Could you check a few things on this drawing? It's one solid part, dimensions in mm from its lowest x, y, z. Give positions to 0.01 mm unless a question says otherwise; leave off trailing zeros. Order: outer loops, then holes, each group sorted by start corner. A loop starts at its lowest first (then second) coordinate and runs counter-clockwise, first axis right, second up. Notation, with made-up numbers: (37.25, 68.25) - (43.25, 68.25) arc R33 ccw to (43.25, 106.25) - close; hole circle Ø5 at (38, -15). An arc over 180 degrees is marked (long way). Return JSON: item names as keys, results as strings.
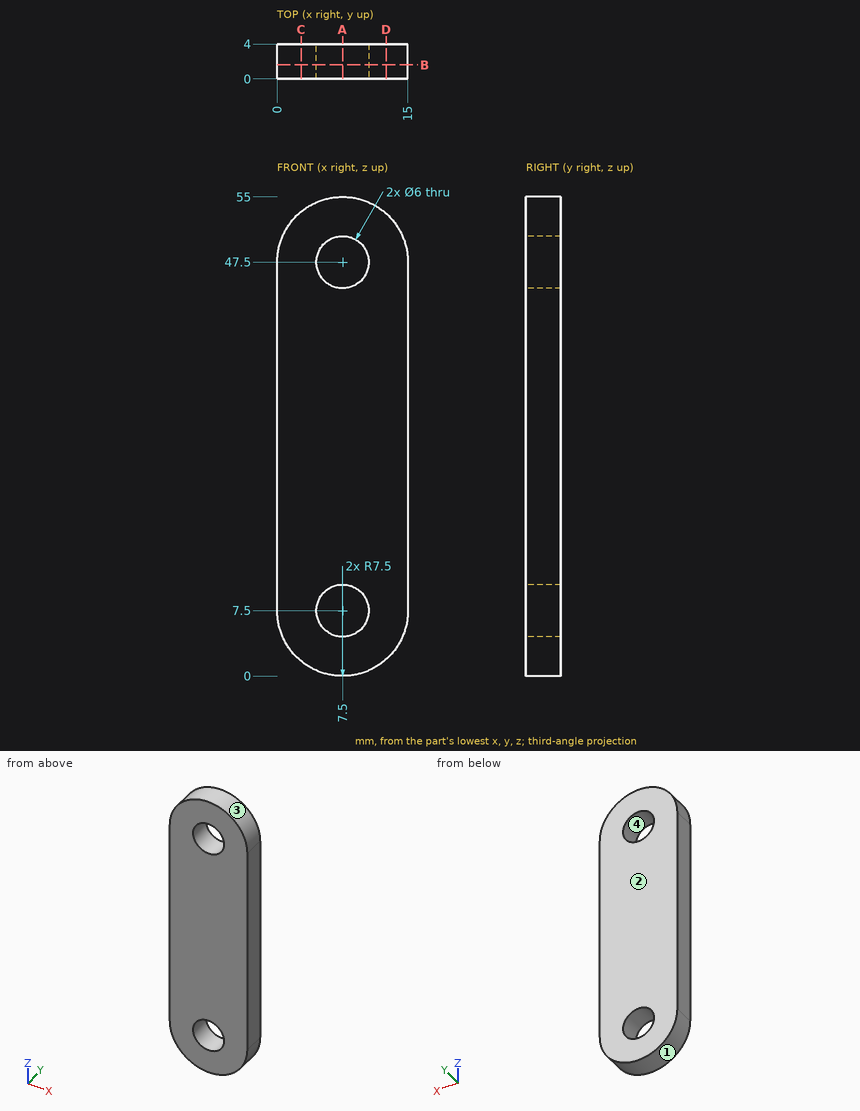
1. Suppose I cut it at D-D (x = 12.5). List the corners of the cut face in (y, z) for me.
Checks:
{"outline": "(0, 1.91) - (4, 1.91) - (4, 53.09) - (0, 53.09) - close"}
2. Suppose I cut it at A-A (x = 7.5). List the corners of the cut face in (y, z) for me, plus the area to 3 significant figures.
Checks:
{"outline": "(0, 0) - (4, 0) - (4, 4.5) - (0, 4.5) - close; (0, 10.5) - (4, 10.5) - (4, 44.5) - (0, 44.5) - close; (0, 50.5) - (4, 50.5) - (4, 55) - (0, 55) - close", "area": "172 mm^2"}
3. If I drill on L1, parallel to Z at x = 7.5, y = 3.15; L2, parallel to Z at x = 10, y = 2.65; L3, parallel to X at y = 3.85, z = 47, over which ranges is the centre line in solid material (lowest first)? Write a range as [from, to].
Checks:
{"L1": "[0, 4.5], [10.5, 44.5], [50.5, 55]", "L2": "[0.43, 5.84], [9.16, 45.84], [49.16, 54.57]", "L3": "[0, 4.54], [10.46, 15]"}
4. Thinking about a two-plate mould opening in Z: for the marked faces 1, 2, 3 and 4, which applies, +Z half, -Z half, draft (parallel to the pull), parting line (faces both ways), or undercut?
Checks:
{"face 1": "-Z half", "face 2": "draft", "face 3": "+Z half", "face 4": "undercut"}
5. Suppose I cut it at C-C (x = 2.75). List the corners of the cut face in (y, z) for me, plus the area to 3 significant figures.
Checks:
{"outline": "(0, 1.7) - (4, 1.7) - (4, 53.3) - (0, 53.3) - close", "area": "206 mm^2"}
6. Suppose I cut it at B-B (y = 1.6). List the corners of the cut face in (x, z) for me, plus the area to 3 significant figures.
Checks:
{"outline": "(0, 7.5) arc R7.5 ccw to (15, 7.5) - (15, 47.5) arc R7.5 ccw to (0, 47.5) - close; hole circle Ø6 at (7.5, 7.5); hole circle Ø6 at (7.5, 47.5)", "area": "720 mm^2"}
